Read the model definition and answer for the solid it produces. Units are mm, in the model's axes. A direction names the side the tool comes from. Coordinates: 2 decimals unless noted, no trailing zeros. Write each loop counter-clockwise with the first axis right and the second up, starting at its lowest first coordinate (ties: lowest second). Pieces come first, ordered by that corner, then holes. Notation, with made-up numbers: M 74.25,21.5 L 93.25,21.5 A13 ccw 93.25,42.5 Z; hole C 37,-27.5 d9. An arc over 180 degrees is marked long. Use a Markdown table: item, result. Add a question column.
Autodesk Inventor part; units mm, degrees
ref_plane "Work Plane1" through (0, 3, -31.5) normal (0, -1, 0) x (1, 0, 0)
ref_plane "YZ Plane" through (0, 0, 0) normal (1, 0, 0) x (0, 1, 0)
ref_plane "XZ Plane" through (0, 0, 0) normal (0, 1, 0) x (-1, 0, 0)
sketch "Sketch1" plane through (0, 0, 0) normal (1, 0, 0) x (0, 1, 0)
  line L0 (0, 0) -> (10.7, 0)
  line L1 (10.7, 0) -> (10.7, -31.5)
  line L2 (10.7, -31.5) -> (0, -31.5)
  line L3 (0, -31.5) -> (0, 0)
  line L4 (0, 0) -> (-20, 0)
  line L5 (-20, 0) -> (-20, -11.5)
  line L6 (-20, -11.5) -> (0, -11.5)
  line L7 (0, -11.5) -> (0, 0)
  line L8 (-20, -6.8471) -> (-12.0113, -11.5)
  dimension "d0" = 10.7
  dimension "d1" = 11.5
  dimension "d2" = 20
  dimension "d4" = 20
extrude "Extrusion1" add sketch "Sketch1" along normal blind 30 contours L0 L1 L2 L3 | L3 L6 L8 L5 L4
sketch "Sketch3" plane through (0, 0, -31.5) normal (0, -1, 0) x (1, 0, 0)
  line L0 (0, 20) -> (0, 0)
  line L1 (0, 0) -> (30, 0)
  line L2 (30, 20) -> (30, 0)
  line L3 (0, 20) -> (30, 20)
  circle A0 centre (15, 8) radius 1.65
  line L4 (15, 0) -> (15, 9.65)
  point P0 (0, 31.5)
  dimension "d10" = 3.3
  dimension "d11" = 8
extrude "Extrusion3" cut sketch "Sketch3" against normal blind 40 contours A0 L4 | L4 A0
ref_plane "Work Plane1" through (0, 3, -31.5) normal (0, -1, 0) x (1, 0, 0)
sketch "Sketch4" plane through (0, 3, -31.5) normal (0, -1, 0) x (1, 0, 0)
  circle A0 centre (15, 8) radius 1.65
  circle A1 centre (20, 8) radius 1.65
  line L0 (15, 4.6514) -> (12.1, 6.3257)
  line L1 (12.1, 6.3257) -> (12.1, 9.6743)
  line L2 (12.1, 9.6743) -> (15, 11.3486)
  line L3 (15, 11.3486) -> (17.9, 9.6743)
  line L4 (17.9, 9.6743) -> (17.9, 6.3257)
  line L5 (17.9, 6.3257) -> (15, 4.6514)
  line L6 (17.9, 6.3257) -> (17.9, 0)
  line L7 (0, 0) -> (30, 0)
  line L8 (12.1, 6.3257) -> (12.1, 0)
  line L9 (17.9, 0) -> (12.1, 0)
  line L10 (0, 0) -> (30, 0)
  line L11 (15, 0) -> (15, 11.3486)
  circle A2 centre (15, 8) radius 1.65
  line L12 (15, 4.6514) -> (17.9, 6.3257)
  line L13 (17.9, 6.3257) -> (17.9, 9.6743)
  line L14 (17.9, 9.6743) -> (15, 11.3486)
  line L15 (15, 11.3486) -> (12.1, 9.6743)
  line L16 (12.1, 9.6743) -> (12.1, 6.3257)
  line L17 (12.1, 6.3257) -> (15, 4.6514)
  line L18 (12.1, 6.3257) -> (12.1, 0)
  line L19 (17.9, 6.3257) -> (17.9, 0)
  line L20 (12.1, 0) -> (17.9, 0)
  point P0 (0, 31.5)
  point P1 (40, 0)
  point P2 (12.1, 0)
  point P3 (17.9, 0)
  dimension "d16" = 5.8
extrude "Extrusion4" cut sketch "Sketch4" against normal blind 3 contours A0 L11 | A0 L11 L3 L4 L5 | L11 A0 | A0 L11 L0 L1 L2 | L11 L7 L8 L0 | L5 L6 L7 L11
sketch "Sketch5" plane through (0, 0, 0) normal (-1, 0, 0) x (0, 0, 1)
  line L0 (0, -20) -> (-6.8471, -20)
  line L1 (0, 10.7) -> (0, -20)
  line L2 (-31.5, 10.7) -> (0, 10.7)
  line L3 (-31.5, 0) -> (-31.5, 10.7)
  line L4 (-11.5, 0) -> (-31.5, 0)
  line L5 (-11.5, -12.0113) -> (-11.5, 0)
  line L6 (-6.8471, -20) -> (-11.5, -12.0113)
  line L7 (-11.5, 10.7) -> (2.3381, 4.9114)
  line L8 (2.3381, 4.9114) -> (0, -20)
  line L9 (-11.5, 0) -> (-11.5, 10.7)
  point P0 (0, 0)
  point P1 (0, 5.8894)
  dimension "d19" = 157.3
  dimension "d20" = 15
extrude "Extrusion5" add sketch "Sketch5" against normal up to surface (30 mm away) contours L1 L7 L8
chamfer "Chamfer1" distance 2 angle 45 1 edges at (15, 4.9114, 2.3381)
extrude "Extrusion6" cut sketch "Sketch5" against normal through all contours L7 L2 L1
properties part number "ESQUINA_RECTA_SUPERIOR" material "Steel, Mild, Welded"
Item 1: Each of these flat-tipped pins is pushed along its axis until it touches: pin 1 (4 mm diameter, centred on x = 10.5, z = -18, fed in from -Y); pin 2 (3.5 mm diameter, centred on x = 13.5, y = -8.5, fed in from -Z); pin 3 (12 mm diameter, centred on x = 7.5, y = -6, fed in from +Z). Where does it stop, or does it pass through?
Item 2: Find section A-A on z = -23.5. Give the vertices of the cut face in (x, y), then the cut area to 3 significant figures.
Item 3: Find section B-B on z = -29. Give the vertices of the cut face in (x, y), then the cut area to 3 significant figures.
Item 4: Find section D-D on y = 8. Give the vertices of the cut face in (x, z), then the cut area to 3 significant figures.
Item 5: Determine the mould class of faces 1 (the flat face through (14.8, 0, -21.6)), 2 (the flat face through (15, 7, -31.5)), 3 (the flat face through (12.1, 4, -27)) for opening direction Y: pulls with the +Y half, pulls with the -Y half, needs draft (parallel to the pull), parting line crosses it, or undercut.
Item 6: Find section C-C on x = 9.5. Give the vertices of the cut face in (y, z).
Item 7: For faces 4 (the flat face through (15, -20, -3)), 5 (the flat face through (17.9, 4, -27)), 6 (the flat face through (15, -6, -11.5)), determine the directions among +Z, -Z, +X, -X, +Y, -Y from which every point of the face is accessible in a straight line to the end or side of a thin tool.
Item 8: Consider probe 1 along X at (y, z) = (1.6, -23.5); probe 2 along X at (y, z) = (5, -27); probe 3 along Y at (x, z) = (21, -25.5). Determine where each line is inside the solid, lowest interval first.
Geometry says:
| question | item | result |
|---|---|---|
| 1 | pin 1 | stops at y = 0 |
| 1 | pin 2 | stops at z = -11.5 |
| 1 | pin 3 | stops at z = 1.88 |
| 2 | outline | M 0,0 L 13.35,0 L 13.35,3 L 12.1,3 L 12.1,6 L 13.35,6 L 13.35,10.7 L 0,10.7 Z; M 16.65,0 L 30,0 L 30,10.7 L 16.65,10.7 L 16.65,6 L 17.9,6 L 17.9,3 L 16.65,3 Z |
| 2 | area | 278 mm2 |
| 3 | outline | M 0,0 L 30,0 L 30,10.7 L 0,10.7 Z; hole M 12.1,3 L 17.9,3 L 17.9,6 L 12.1,6 Z |
| 3 | area | 304 mm2 |
| 4 | outline | M 0,-31.5 L 30,-31.5 L 30,-5.05 L 0,-5.05 Z; hole C 15,-23.5 d3.3 |
| 4 | area | 785 mm2 |
| 5 | face 1 | pulls with the -Y half |
| 5 | face 2 | needs draft |
| 5 | face 3 | undercut |
| 6 | outline | M -20,-6.85 L -12.01,-11.5 L 0,-11.5 L 0,-31.5 L 10.7,-31.5 L 10.7,-11.5 L 5.68,0.49 L 2.92,2.15 L -20,0 Z |
| 7 | face 4 | +Z, -Z, +X, -X, -Y |
| 7 | face 5 | -Z |
| 7 | face 6 | -Z, +X, -X, -Y |
| 8 | probe 1 | x = 0 to 13.35, 16.65 to 30 |
| 8 | probe 2 | x = 0 to 12.1, 17.9 to 30 |
| 8 | probe 3 | y = 0 to 10.7 |
